Print and shaded views of the part. All mm, measured from the part's lowest x, y and z. Give positions to 0.01 mm unless a question says otherwise; leave off trailing zeros. Loops run counter-clockwise (first coordinate to the right, second up) from the corner with the lowest first, then second, coordinate; pieces in that order, holes last. Notation, with made-up numbers: M -17.75,15.25 L -2.75,15.25 A11 cw -2.75,22.25 Z; hole C 1.5,65.25 d9. An arc over 180 degrees is marked long. Answer as CSV lines item,"result".
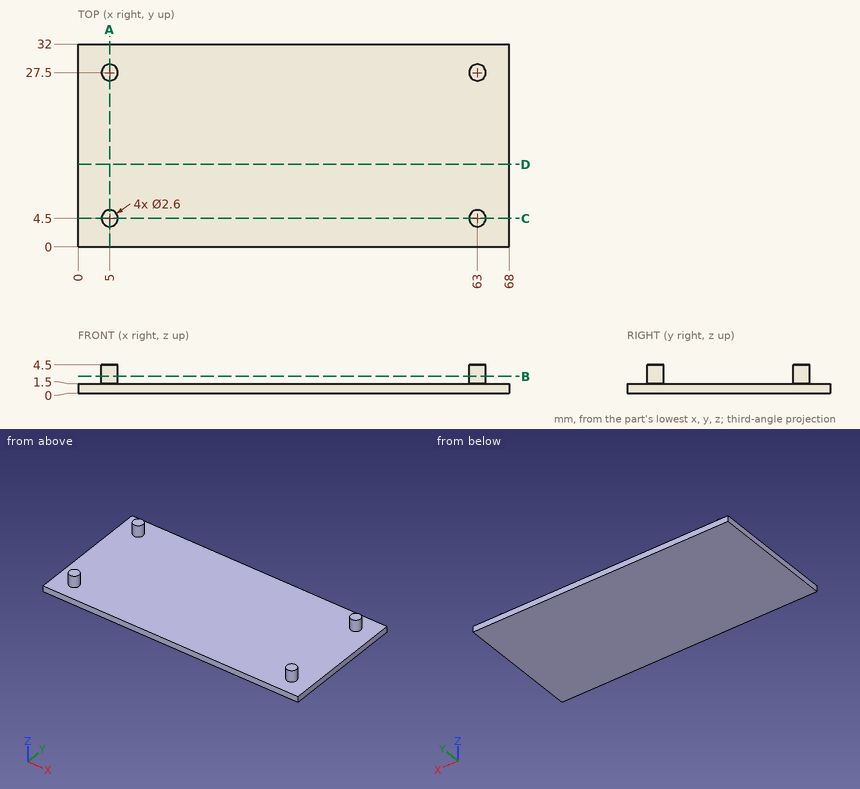
Q1. Cut at A-A (x = 5). Write the cut outline in (y, z).
Solution:
outline,"M 0,0 L 32,0 L 32,1.5 L 28.8,1.5 L 28.8,4.5 L 26.2,4.5 L 26.2,1.5 L 5.8,1.5 L 5.8,4.5 L 3.2,4.5 L 3.2,1.5 L 0,1.5 Z"
Q2. Cut at D-D (y = 13). Write the cut outline in (x, z), and give its area (3 significant figures).
Solution:
outline,"M 0,0 L 68,0 L 68,1.5 L 0,1.5 Z"
area,"102 mm²"
Q3. Pin check, flat tip, straight feed: P1, Ø2, axis at x = 58, y = 12, coming from the +Z side. Stop position of the tip, or through.
Solution:
P1,"stops at z = 1.5"
Q4. Wall check: line 1 (Z direction, x = 27.5, y = 22); line 2 (X direction, y = 28, z = 2.05); line 3 (X direction, y = 28.5, z = 3.15). Give the ranges that are in metal, low to high. Write a range as [from, to].
Solution:
line 1,"z = [0, 1.5]"
line 2,"x = [3.8, 6.2], [61.8, 64.2]"
line 3,"x = [4.17, 5.83], [62.17, 63.83]"
Q5. Cut at B-B (z = 2.7). Write the cut outline in (x, y), and give its area (3 significant figures).
Solution:
outline,"C 5,4.5 d2.6; C 5,27.5 d2.6; C 63,4.5 d2.6; C 63,27.5 d2.6"
area,"21.2 mm²"
Q6. Cut at C-C (y = 4.5). Write the cut outline in (x, z), and give its area (3 significant figures).
Solution:
outline,"M 0,0 L 68,0 L 68,1.5 L 64.3,1.5 L 64.3,4.5 L 61.7,4.5 L 61.7,1.5 L 6.3,1.5 L 6.3,4.5 L 3.7,4.5 L 3.7,1.5 L 0,1.5 Z"
area,"118 mm²"
